```python
from build123d import *

# Parameters (mm, degrees)
BOSS_EXTRUDE1_DEPTH   = 3.175
M3_CLEARANCE_HOLE1_D  = 3.4
FILLET1_R             = 10
F_8_CLEARANCE_HOLE1_D = 4.4958
LPATTERN1_COUNT       = 5
LPATTERN1_PITCH       = 100


with BuildPart() as part:
    # Sketch1 → Boss-Extrude1 (new body)
    with BuildSketch(Plane(origin=(0, 0, 0), x_dir=(0, 0, -1), z_dir=(1, 0, 0))):
        Polygon((0, 0), (0, 40), (546, 40), (546, 20), (50, 0), align=None)
    extrude(amount=BOSS_EXTRUDE1_DEPTH)

    # M3 Clearance Hole1 (through all)
    with Locations(Plane(origin=(3.175, 33, -26), x_dir=(0, 0, 1), z_dir=(1, 0, 0))):
        with Locations((0, 0), (20, 0), (0, 20), (20, 20)):
            Hole(M3_CLEARANCE_HOLE1_D / 2)

    # Fillet1
    # the kernel refuses this fillet: 10 mm, written as the material it takes off along each edge
    with BuildSketch(Plane(origin=(-25, 0, 0), x_dir=(0, 1, 0), z_dir=(1, 0, 0))) as fillet1_piece_1:
        with BuildLine():
            CenterArc((FILLET1_R, -FILLET1_R), FILLET1_R, 90, 90)
            Line((0, -FILLET1_R), (0, 0))
            Line((0, 0), (FILLET1_R, 0))
        make_face()
    extrude(amount=53.175, mode=Mode.SUBTRACT)
    with BuildSketch(Plane(origin=(-24.012251111, 20, -546), x_dir=(0, -0.04028984011081184, 0.9991880347481376), z_dir=(1, 0, 0))) as fillet1_piece_2:
        with BuildLine():
            CenterArc((FILLET1_R * 0.96049004443, -FILLET1_R), FILLET1_R, 90, 87.690937211)
            Line((-FILLET1_R * 0.0386979903181, -FILLET1_R * 0.959710159889), (0, 0))
            Line((0, 0), (FILLET1_R * 0.96049004443, 0))
        make_face()
    extrude(amount=51.199502222, mode=Mode.SUBTRACT)
    with BuildSketch(Plane(origin=(-0.503827547, 0, -50), x_dir=(0, 0, 1), z_dir=(1, 0, 0))) as fillet1_piece_3:
        with BuildLine():
            CenterArc((FILLET1_R * 0.0201531018646, -FILLET1_R), FILLET1_R, 90, 2.309062789)
            Line((-FILLET1_R * 0.0201367382462, -FILLET1_R * 0.000811965251862), (0, 0))
            Line((0, 0), (FILLET1_R * 0.0201531018646, 0))
        make_face()
    extrude(amount=4.182655093, mode=Mode.SUBTRACT)

    # #8 Clearance Hole1 (through all)
    with Locations(Plane(origin=(3.175, 30.475, -496), x_dir=(0, 0, 1), z_dir=(1, 0, 0))):
        with Locations((0, 0)):
            f_8_clearance_hole1 = Hole(F_8_CLEARANCE_HOLE1_D / 2)

    # LPattern1: #8 Clearance Hole1 ×5
    with Locations(*[(0, 0, i * LPATTERN1_PITCH) for i in range(1, LPATTERN1_COUNT)]):
        add(f_8_clearance_hole1, mode=Mode.SUBTRACT)


solid = part.part
```
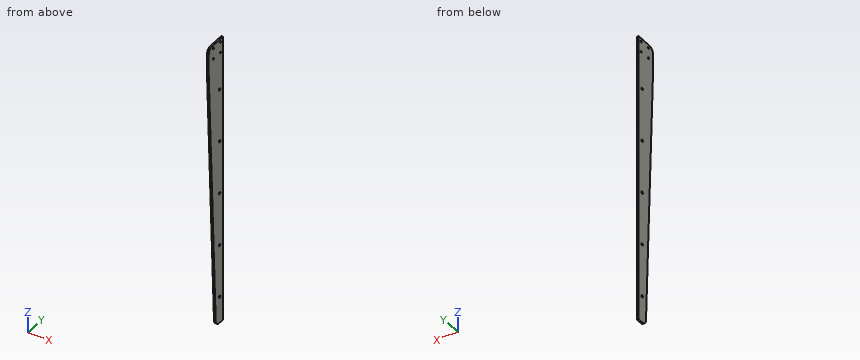
Here's how the part is built. I have some questions about the finished solid (model axes, mm). Give positions to 0.01 mm unless a question says otherwise; leave off trailing zeros. Write each loop counter-clockwise with the first axis right and the second up, starting at its lowest first coordinate (ties: lowest second). Pieces come first, ordered by that corner, then holes. Notation, with made-up numbers: M -29.75,29.25 L -15.75,29.25 A22 cw -15.75,66.25 Z; hole C 76,56 d7. An arc over 180 degrees is marked long. Put each result on its own line as item: value. Start each with the question number.
Item 1: If we section it at C-C, the plane z = -146.5: Write out the boundary of the cut face in (x, y) (3 decimals), then the cut area to 3 significant figures.
Item 2: If we section it at A-A, the plane x = 1.5: Count the separate pieces of the cut face and the enclosed holes in it, then the cut area to 3 significant figures.
Item 3: Will these pins go through, and if not, where does the flat tip stop? pin 1 (7 mm diameter, centred on y = 30.475, z = -96, fed in from -X); pin 2 (1 mm diameter, centred on x = 2.5, y = 27, fed in from -Z); pin 3 (1 mm diameter, centred on x = 1, z = -368.5, fed in from -Y).
Item 4: I need wall thicknesses on L1, parallel to Z at x = 1.15, y = 33; L2, parallel to Y at x = 0.85, z = -26; L3, parallel to Z at x = 0.55, y = 29.5. Which ranges of each line are inside material? Lowest first, please. Write a range as from..to.
Item 5: If we section it at B-B, the plane z = -506: Write out the boundary of the cut face in (x, y) (3 decimals).
Values:
1. outline: M 0,3.891 L 3.175,3.891 L 3.175,40 L 0,40 Z
1. area: 115 mm²
2. separate pieces: 1
2. enclosed holes: 9
2. area: 16,700 mm²
3. pin 1: x = 0
3. pin 2: z = -545.78
3. pin 3: y = 12.82
4. L1: -546..-27.7, -24.3..-7.7, -4.3..0
4. L2: 0..11.3, 14.7..31.3, 34.7..40
4. L3: -546..-498.03, -493.97..-398.03, -393.97..-298.03, -293.97..-198.03, -193.97..-98.03, -93.97..0
5. outline: M 0,18.387 L 3.175,18.387 L 3.175,40 L 0,40 Z
